For this review, use the dimensioned drawing (mm, ordinates from the lowest corner) and the shaded views. A direction names the side the tool comes from. Give positions to 0.01 mm unless a question says otherwise; leave off trailing zeros. Loops run counter-clockwise (first coordinate to the right, second up) from the corner with the lowest first, then second, coordinate; pieces in that order, holes last. Notation, with made-up numbers: (53.5, 32.5) - (102.5, 32.5) arc R22 ccw to (102.5, 59.5) - close; hole circle Ø9 at (-29.75, -16). An arc over 180 degrees is marked (long way). Write each question's results on one line, items separated by ' | '.
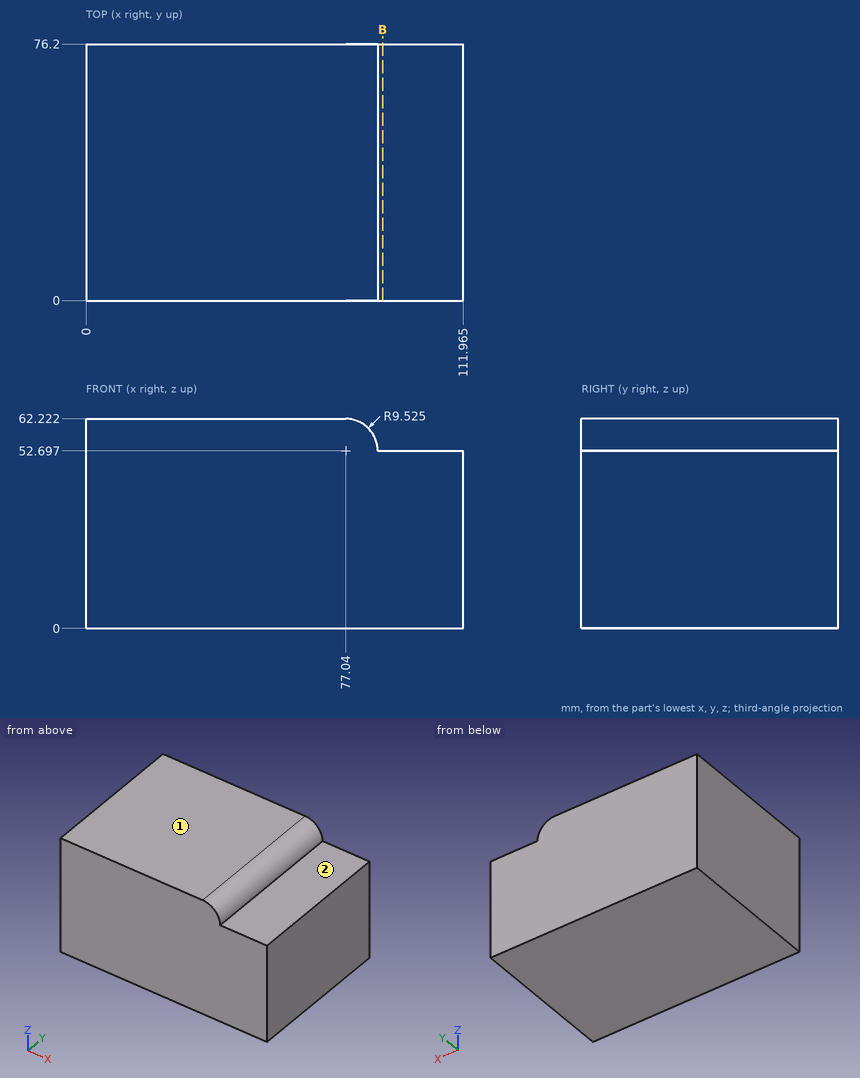
Item 1: Wall thickness on probe 1 along Z at (x, y) = (94.5, 73): over which ranges is the line inside the solid? List them lowest first.
Output values:
probe 1: z = 0 to 52.7
Item 2: Clearance check with a flat-ended pin moving along its axis: P1, Ø12.5, axis at x = 93.5, y = 31.5, coming from the +Z side. State where the tip first meets the part, or that it passes through.
Output values:
P1: stops at z = 52.7
Item 3: We need section B-B on x = 88. Give the boundary of the cut face in (y, z), then the cut area to 3 significant figures.
Output values:
outline: (0, 0) - (76.2, 0) - (76.2, 52.7) - (0, 52.7) - close | area: 4,020 mm²
Item 4: Tool access review of the marked faces 1 and 2: name each direction out of +Z, -Z, +X, -X, +Y, -Y from which nothing blocks a thin tool from reaching the whole face with its end or side.
Output values:
face 1: +Z, +X, -X, +Y, -Y | face 2: +Z, +X, +Y, -Y
